Part model, mm, in its own coordinate system. Give positions to 0.01 mm unless a question says otherwise; leave off trailing zeros. Write each loop counter-clockwise with the first axis right and the second up, starting at its lowest first coordinate (ties: lowest second). Pieces come first, ordered by that corner, then holes.
Autodesk Inventor part; units mm, degrees
ref_plane "YZ Plane" through (0, 0, 0) normal (1, 0, 0) x (0, 1, 0)
ref_plane "XZ Plane" through (0, 0, 0) normal (0, 1, 0) x (-1, 0, 0)
ref_plane "XY Plane" through (0, 0, 0) normal (0, 0, 1) x (1, 0, 0)
sketch "Skizze1" plane through (0, 0, 0) normal (0, 0, 1) x (1, 0, 0)
  line L0 (0, -1.9) -> (0, 11.4) construction
  line L1 (-7.5, 0) -> (7.5, 0)
  line L2 (7.5, 0) -> (7.5, 9.5)
  line L3 (7.5, 9.5) -> (-7.5, 9.5)
  line L4 (-7.5, 9.5) -> (-7.5, 0)
  circle A0 centre (-7.5, 6.5) radius 1.5
  line L5 (-12.6, 0) -> (12.6, 0)
  line L6 (-4.5, 6.5) -> (-7.5, 6.5) construction
  line L7 (-4.5, 7) -> (-7.5, 7)
  line L8 (-7.5, 6) -> (-4.5, 6)
  arc A1 (-4.5, 6) -> (-4.5, 7) centre (-4.5, 6.5) ccw
  arc A2 (-7.5, 7) -> (-7.5, 6) centre (-7.5, 6.5) ccw
  circle A3 centre (-4.5, 6.5) radius 1
  circle A4 centre (7.5, 6.5) radius 1.5
  line L9 (4.5, 7) -> (7.5, 7)
  line L10 (7.5, 6) -> (4.5, 6)
  arc A5 (4.5, 7) -> (4.5, 6) centre (4.5, 6.5) ccw
  circle A6 centre (4.5, 6.5) radius 1
  point P0 (0, 0)
  point P1 (0, 0)
  point P2 (-7.5, 8)
  point P3 (-7.5, 5)
  point P4 (-6, 6.5)
  point P5 (6, 6.5)
  point P6 (-6.0858, 7)
  point P7 (-5.366, 7)
  point P8 (-5.366, 6)
  point P9 (-6.0858, 6)
  point P10 (7.5, 5)
  point P11 (6.0858, 6)
  point P12 (5.366, 6)
  point P13 (5.366, 7)
  point P14 (6.0858, 7)
  point P15 (7.5, 8)
  dimension "d2" = 3
  dimension "d0" = 15
  dimension "d1" = 9.5
  dimension "d3" = 3
  dimension "d6" = 1
  dimension "d7" = 2
extrude "Extrusion1" add sketch "Skizze1" along normal blind 1000 contours L4 A0 L8 A3 L7 L3 L2 A4 L9 A6 L10 L1
sketch "Skizze2" plane through (-7.5, 9.5, 1000) normal (0, 1, 0) x (1, 0, 0)
  line L0 (-3, 1000) -> (18, 1000)
  line L1 (7.5, 1200) -> (7.5, -200)
  circle A0 centre (7.5, 980) radius 3
  circle A1 centre (7.5, 980) radius 1.75
  point P0 (7.5, 1000)
  dimension "d8" = 6
  dimension "d9" = 3.5
  dimension "d10" = 20
extrude "Extrusion2" cut sketch "Skizze2" against normal blind 6
extrude "Extrusion3" cut sketch "Skizze2" against normal blind 15 contours A1 L1 | L1 A1
chamfer "Fase1" distance 1 angle 45 1 edges at (-3, 9.5, 20)
pattern_linear "Rechteckige Anordnung1" count 25 spacing 40 along (0, 0, 1) of "Extrusion2", "Extrusion3", "Fase1"
equation "\"d4\" = Raillänge"
equation "\"Raillänge\" = 1000"
properties part number "MGN15 Linear Rail 1000mm"
1) Wall check: L1, parallel to X at y = 2.15, z = 740; L2, parallel to Y at x = 5.5, z = 565.5; L3, parallel to Y at x = 4, z = 262.5. Give the ranges that are in metal, low to high.
Answers follow:
L1: x = -7.5 to -1.75, 1.75 to 7.5
L2: y = 0 to 6, 7 to 9.5
L3: y = 0 to 5.63, 7.37 to 9.5
2) Pin check, flat tips, straight feed: pin 1 Ø3 at (x, z) = (1, 941.5) entering from +Y; pin 2 Ø1.2 at (x, y) = (-4.5, 6.5) entering from +Z (3 decimals); pin 3 Ø3 at (x, z) = (1, 860.5) entering from +Y; pin 4 Ø3 at (x, z) = (0.5, 741.5) entering from +Y. Stop position of each tip, or through.
Answers follow:
pin 1: stops at y = 8.8
pin 2: passes through
pin 3: stops at y = 3.5
pin 4: stops at y = 8.58
3) Saw through at B-B, the plane z = 917. Write the cut outline in (x, y), then the cut area to 3 significant figures.
Answers follow:
outline: (-7.5, 0) - (7.5, 0) - (7.5, 5) arc R1.5 cw to (6.09, 6) - (5.37, 6) arc R1 cw (long way) to (5.37, 7) - (6.09, 7) arc R1.5 cw to (7.5, 8) - (7.5, 9.5) - (-7.5, 9.5) - (-7.5, 8) arc R1.5 cw to (-6.09, 7) - (-5.37, 7) arc R1 cw (long way) to (-5.37, 6) - (-6.09, 6) arc R1.5 cw to (-7.5, 5) - close
area: 128 mm2
4) Saw through at A-A, the plane y = 1.5. Count the separate pieces of the cut face and the enclosed holes in it, then the cut area to 3 significant figures.
Answers follow:
separate pieces: 1
enclosed holes: 25
area: 14,800 mm2
